Design review of the part built by this model. Coordinates are the model's own, in mm. Coordinates: 2 decimals unless noted, no trailing zeros. Write each loop counter-clockwise with the first axis right and the second up, starting at its lowest first coordinate (ties: lowest second). Pieces come first, ordered by that corner, then holes. Notation, with made-up numbers: (-18.75, 0) -> (18.25, 0) arc R28 ccw to (18.25, 18) -> close; hole circle Ø2 at (55.5, 7). An arc over 180 degrees is marked (long way). Answer in a Markdown table with one row per item. Add a question column.
Item 1: Clearance check with a flat-ended pin moving along its axis: P1, Ø5, axis at y = 17, z = 48.5, coming from the +X side. State where the tip first meets the part, or that it passes through.
Item 2: Take a section at C-C, the plane z = 41. Write out the cut boundary in (x, y).
Item 3: Take a section at A-A, the plane y = 24. Write out the cut boundary in (x, z), and give its area (3 significant figures).
Item 4: To check wall thickness, follow line 1 (X direction, y = -12.5, z = 50); line 2 (X direction, y = -9, z = 58). State the ranges of each line that lie inside material, in increasing order.
Item 5: Take a section at B-B, the plane z = 53. Write out the cut boundary in (x, y), and give its area (3 significant figures).
from build123d import *

# Parameters (mm, degrees)
F0_W     = 127
F0_H     = 76.2
F1_DEPTH = 0.762
F3_DEPTH = 76.2


with BuildPart() as f1:
    # F0 (on Top) → F1 (new body)
    with BuildSketch(Plane.XY):
        with Locations((-0.68152, 2.694871)):
            Rectangle(F0_W, F0_H)
    extrude(amount=F1_DEPTH)

    # F2 (on face) → F3 (join)
    with BuildSketch(Plane.XZ.offset(35.405129)):
        Polygon((-64.18152, 0.762), (62.81848, 0.762), (62.81848, 16.655238), (55.19848, 63.5), (-56.56152, 63.5), (-64.18152, 16.655238), align=None)
    extrude(amount=-F3_DEPTH)


solid = f1.part
Answers:
| question | item | result |
|---|---|---|
| 1 | P1 | stops at x = 58.05 |
| 2 | outline | (-60.22, -35.41) -> (58.86, -35.41) -> (58.86, 40.79) -> (-60.22, 40.79) -> close |
| 3 | outline | (-64.18, 0) -> (62.82, 0) -> (62.82, 16.66) -> (55.2, 63.5) -> (-56.56, 63.5) -> (-64.18, 16.66) -> close |
| 3 | area | 7,710 mm^2 |
| 4 | line 1 | x = -58.76 to 57.39 |
| 4 | line 2 | x = -57.46 to 56.09 |
| 5 | outline | (-58.27, -35.41) -> (56.91, -35.41) -> (56.91, 40.79) -> (-58.27, 40.79) -> close |
| 5 | area | 8,780 mm^2 |
